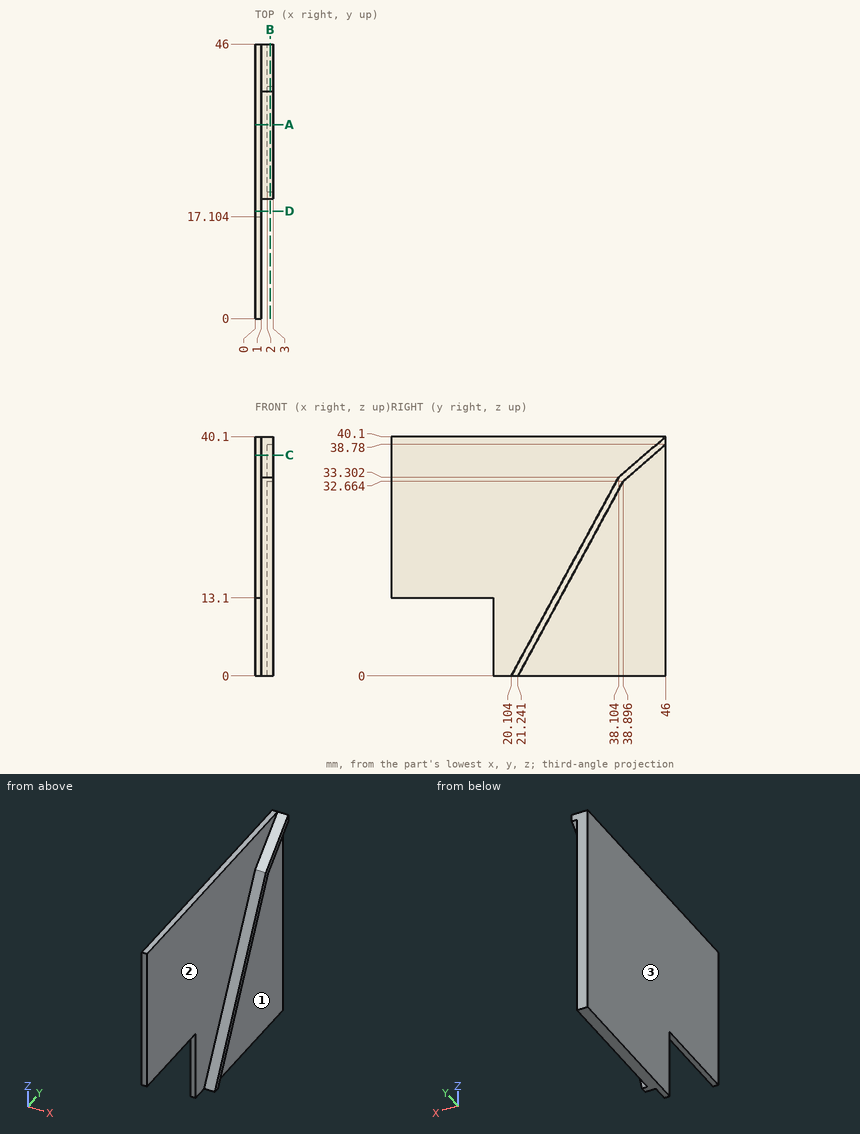
Source: three-view drawing plus pictorial views. Frame: mm from the lowest corner of the part. A direction names the side the tool comes from. Coordinates: 2 decimals unless noted, no trailing zeros. Loops run counter-clockwise (first coordinate to the right, second up) from the corner with the lowest first, then second, coordinate; pieces in that order, holes last. Notation, with made-up numbers: (5, -35.5) - (61, -35.5) arc R20 ccw to (61, -4.5) - close; hole circle Ø6 at (1.25, 54.5). An arc over 180 degrees is marked (long way). One line per question, with ' | ' between items.
1) Section D-D, the plane y = 18. Return loops of the section in (x, z).
Report:
outline: (0, 0) - (1, 0) - (1, 40.1) - (0, 40.1) - close
2) Section B-B, the plane x = 2.5. Return loops of the section in (y, z).
Report:
outline: (20.1, 0) - (21.24, 0) - (38.9, 32.66) - (46, 38.78) - (46, 40.1) - (38.1, 33.3) - close
3) Section A-A, the plane y = 32.5. Return loops of the section in (x, z).
Report:
outline: (0, 0) - (2, 0) - (2, 20.83) - (3, 20.83) - (3, 22.93) - (1, 22.93) - (1, 40.1) - (0, 40.1) - close
4) Set-up query: the marked faces 1, 2 and 3. Return all of +Z, -Z, +X, -X, +Y, -Y with unobstructed straight access to the full face (end or side cutting, diameter ignored); none if empty.
Report:
face 1: -Z, +X, +Y | face 2: +Z, +X, -Y | face 3: +Z, -Z, -X, +Y, -Y
5) Section C-C, the plane z = 37. Return loops of the section in (x, y).
Report:
outline: (0, 0) - (1, 0) - (1, 42.4) - (3, 42.4) - (3, 43.93) - (2, 43.93) - (2, 46) - (0, 46) - close
6) First-contact query: P1, Ø4, axis at y = 25.5, z = 26.5, coming from the +X side; P2, Ø0.5, axis at x = 0.5, z = 6, coming from the -Y side. Flat tips, straight axial feed; report the tip coordinate or a pass-through.
Report:
P1: stops at x = 1 | P2: stops at y = 17.1
7) Line query: line 1 along X through (y, z) = (7.5, 34); line 2 along X through (y, z) = (35, 17); line 3 along Y through (x, z) = (0.25, 2). Output: solid intervals per line, ascending.
Report:
line 1: x = 0 to 1 | line 2: x = 0 to 2 | line 3: y = 17.1 to 46
